from build123d import *

# Parameters (mm, degrees)
SKETCH2_W                     = 342.9
SKETCH2_H                     = 431.8
BASE_DEPTH                    = 25.4
CUT_EXTRUDE3_REACH            = 27.4
NC_POCKET_DEPTH               = 16.51
FILLET9_R                     = 6.35
FILLET6_R                     = 6.35
CBORE_FOR_M4_SHCS1_AT_2_COUNT = 2
CBORE_FOR_M4_SHCS1_AT_2_PITCH = 192.024
CBORE_FOR_M4_SHCS1_AT_3_COUNT = 2
CBORE_FOR_M4_SHCS1_AT_3_PITCH = 313.675937134
CBORE_FOR_M4_SHCS1_AT_4_COUNT = 2
CBORE_FOR_M4_SHCS1_AT_4_PITCH = 253.241439295
CBORE_FOR_M4_SHCS1_AT_5_COUNT = 2
CBORE_FOR_M4_SHCS1_AT_5_PITCH = 135.860323862
SKETCH18_R                    = 7.1755
CUT_EXTRUDE4_DEPTH            = 1.016
F_3_8_16_TAPPED_HOLE1_D       = 7.9375
F_3_8_16_TAPPED_HOLE1_DEPTH   = 27.94
F_3_8_16_TAPPED_HOLE1_TIP     = 2.384665582
F_3_8_16_TAPPED_HOLE2_D       = 7.9375
F_3_8_16_TAPPED_HOLE2_DEPTH   = 20.32
F_3_8_16_TAPPED_HOLE2_TIP     = 2.384665582
CUT_EXTRUDE5_REACH            = 10.89
FILLET1_R                     = 6.35
FILLET2_R                     = 6.35
CHAMFER1_SIZE                 = 0.508
SKETCH21_W                    = 6.35
SKETCH21_H                    = 431.8
CUT_EXTRUDE6_DEPTH            = 6.35
SKETCH22_W                    = 6.35
SKETCH22_H                    = 431.8
CUT_EXTRUDE7_DEPTH            = 3.81
SKETCH23_W                    = 33.02
SKETCH23_H                    = 48.26
CUT_EXTRUDE8_DEPTH            = 10.16
FILLET10_R                    = 6.35


with BuildPart() as part:
    # Sketch2 → Base (new body)
    with BuildSketch(Plane(origin=(0, 0, 0), x_dir=(0, 0, -1), z_dir=(1, 0, 0))):
        with Locations((-44.038996764, -78.624919094)):
            Rectangle(SKETCH2_W, SKETCH2_H)
    extrude(amount=BASE_DEPTH)

    # Sketch3 → Cut-Extrude3 (cut, up to next)
    with BuildSketch(Plane(origin=(0, 0, 0), x_dir=(0, 0, -1), z_dir=(1, 0, 0)), mode=Mode.PRIVATE) as cut_extrude3_sk1:
        Polygon((-164.688996764, -25.919919094), (-164.688996764, -229.119919094), (51.211003236, -229.119919094), (51.211003236, -146.950919094), (25.811003236, -146.950919094), (25.811003236, -25.919919094), align=None)
    cut_extrude3_tool1 = extrude(cut_extrude3_sk1.sketch, amount=CUT_EXTRUDE3_REACH, mode=Mode.PRIVATE) & part.part
    add(cut_extrude3_tool1.solids().sort_by_distance((0, -130.615794, 63.91645))[0], mode=Mode.SUBTRACT)

    # Sketch4 → NC pocket (cut)
    with BuildSketch(Plane(origin=(0, 0, 0), x_dir=(0, 0, -1), z_dir=(1, 0, 0))):
        Polygon((19.461003236, -18.299919094), (-158.338996764, -18.299919094), (-158.338996764, -25.919919094), (-164.688996764, -25.919919094), (-164.688996764, -12.583714933), (-164.688996764, -3.059919094), (-215.488996764, -3.059919094), (-215.488996764, 25.515080906), (-164.688996764, 25.515080906), (-164.688996764, 86.475080906), (-215.488996764, 86.475080906), (-215.488996764, 90.285080906), (-215.488996764, 137.275080906), (-202.788996764, 137.275080906), (51.211003236, 137.275080906), (51.211003236, -15.124919094), (51.211003236, -53.859919094), (79.405003236, -82.053919094), (51.211003236, -110.247919094), (51.211003236, -136.155919094), (51.211003236, -146.950919094), (44.861003236, -146.950919094), (44.861003236, -139.330919094), (25.811003236, -139.330919094), (25.811003236, -25.919919094), (19.461003236, -25.919919094), align=None)
    extrude(amount=NC_POCKET_DEPTH, mode=Mode.SUBTRACT)

    # Fillet9
    fillet9_edges = [part.edges().sort_by_distance(p)[0] for p in [
        (8.255, -53.859919094, -51.211003236),
        (8.255, -110.247919094, -51.211003236),
    ]]
    fillet(fillet9_edges, radius=FILLET9_R)

    # Fillet6
    fillet6_edges = [part.edges().sort_by_distance(p)[0] for p in [
        (8.255, -82.053919094, -79.405003236),
    ]]
    fillet(fillet6_edges, radius=FILLET6_R)

    # Sketch10 → CBORE for M4 SHCS1 (revolve, cut)
    with BuildSketch(Plane(origin=(25.4, 124.575080906, 151.988996764), x_dir=(0, 0, -1), z_dir=(0, 1, 0))):
        Polygon((0, 0), (0, 8.89), (2.15, 8.89), (2.15, 4), (4, 4), (4, 1), (5, 0), align=None)
    cbore_for_m4_shcs1 = revolve(axis=Axis((31.75, 124.575080906, 151.988996764), (-1, 0, 0)), mode=Mode.SUBTRACT)

    # CBORE for M4 SHCS1 at 2: CBORE for M4 SHCS1 ×2
    with Locations(*[(0, 0, -i * CBORE_FOR_M4_SHCS1_AT_2_PITCH) for i in range(1, CBORE_FOR_M4_SHCS1_AT_2_COUNT)]):
        add(cbore_for_m4_shcs1, mode=Mode.SUBTRACT)

    # CBORE for M4 SHCS1 at 3: CBORE for M4 SHCS1 ×2
    with Locations(*[Vector(0, -0.790723708, -0.612173193) * (i * CBORE_FOR_M4_SHCS1_AT_3_PITCH) for i in range(1, CBORE_FOR_M4_SHCS1_AT_3_COUNT)]):
        add(cbore_for_m4_shcs1, mode=Mode.SUBTRACT)

    # CBORE for M4 SHCS1 at 4: CBORE for M4 SHCS1 ×2
    with Locations(*[Vector(0, -0.651947013, -0.758264526) * (i * CBORE_FOR_M4_SHCS1_AT_4_PITCH) for i in range(1, CBORE_FOR_M4_SHCS1_AT_4_COUNT)]):
        add(cbore_for_m4_shcs1, mode=Mode.SUBTRACT)

    # CBORE for M4 SHCS1 at 5: CBORE for M4 SHCS1 ×2
    with Locations(*[Vector(0, -0.934783581, -0.355217761) * (i * CBORE_FOR_M4_SHCS1_AT_5_PITCH) for i in range(1, CBORE_FOR_M4_SHCS1_AT_5_COUNT)]):
        add(cbore_for_m4_shcs1, mode=Mode.SUBTRACT)

    # Sketch18 → Cut-Extrude4 (cut)
    with BuildSketch(Plane.ZY.offset(-16.51)):
        with Locations((-40.035003236, 124.575080906)):
            Circle(SKETCH18_R)
        with Locations((151.988996764, 124.575080906)):
            Circle(SKETCH18_R)
        with Locations((103.728996764, -2.424919094)):
            Circle(SKETCH18_R)
        with Locations((-40.035003236, -40.524919094)):
            Circle(SKETCH18_R)
        with Locations((-40.035003236, -123.455919094)):
            Circle(SKETCH18_R)
    extrude(amount=-CUT_EXTRUDE4_DEPTH, mode=Mode.SUBTRACT)

    # 3/8-16 Tapped Hole1
    with Locations(Plane(origin=(12.7, -294.524919094, -70.261003236), x_dir=(0, 0, -1), z_dir=(0, -1, 0))):
        with Locations((0, 0), (-114.3, 0), (-228.6, 0)):
            Hole(F_3_8_16_TAPPED_HOLE1_D / 2, depth=F_3_8_16_TAPPED_HOLE1_DEPTH)
            with Locations((0, 0, -(F_3_8_16_TAPPED_HOLE1_DEPTH + F_3_8_16_TAPPED_HOLE1_TIP / 2))):  # 118° drill point
                Cone(0, F_3_8_16_TAPPED_HOLE1_D / 2, F_3_8_16_TAPPED_HOLE1_TIP, mode=Mode.SUBTRACT)

    # 3/8-16 Tapped Hole2
    with Locations(Plane.ZY):
        with Locations((188.501496764, -220.864919094), (188.501496764, -162.444919094), (-100.423503236, -220.864919094), (-100.423503236, -162.444919094)):
            Hole(F_3_8_16_TAPPED_HOLE2_D / 2, depth=F_3_8_16_TAPPED_HOLE2_DEPTH)
            with Locations((0, 0, -(F_3_8_16_TAPPED_HOLE2_DEPTH + F_3_8_16_TAPPED_HOLE2_TIP / 2))):  # 118° drill point
                Cone(0, F_3_8_16_TAPPED_HOLE2_D / 2, F_3_8_16_TAPPED_HOLE2_TIP, mode=Mode.SUBTRACT)

    # Sketch20 → Cut-Extrude5 (cut, up to next)
    with BuildSketch(Plane.ZY.offset(-16.51), mode=Mode.PRIVATE) as cut_extrude5_sk1:
        Polygon((-51.211003236, -53.859919094), (-25.811003236, -53.859919094), (-25.811003236, -110.247919094), (-51.211003236, -110.247919094), (-79.405003236, -82.053919094), align=None)
    cut_extrude5_tool1 = extrude(cut_extrude5_sk1.sketch, amount=-CUT_EXTRUDE5_REACH, mode=Mode.PRIVATE) & part.part
    add(cut_extrude5_tool1.solids().sort_by_distance((16.51, -82.053919, -46.398071))[0], mode=Mode.SUBTRACT)

    # Fillet1
    fillet1_edges = [part.edges().sort_by_distance(p)[0] for p in [
        (20.955, -25.919919094, 164.688996764),
        (12.7, -229.119919094, 164.688996764),
        (12.7, -229.119919094, -51.211003236),
        (20.955, -146.950919094, -51.211003236),
        (20.955, -25.919919094, -25.811003236),
    ]]
    fillet(fillet1_edges, radius=FILLET1_R)

    # Fillet2
    fillet2_edges = [part.edges().sort_by_distance(p)[0] for p in [
        (20.955, -82.053919094, -79.405003236),
        (20.955, -110.247919094, -51.211003236),
        (20.955, -53.859919094, -51.211003236),
    ]]
    fillet(fillet2_edges, radius=FILLET2_R)

    # Chamfer1
    chamfer1_edges = [part.edges().sort_by_distance(p)[0] for p in [
        (12.7, -146.950919094, -25.811003236),
        (20.955, -53.859919094, -25.811003236),
        (20.955, -110.247919094, -25.811003236),
        (8.255, 86.475080906, 215.488996764),
        (8.255, 86.475080906, 164.688996764),
        (8.255, 25.515080906, 164.688996764),
        (8.255, 25.515080906, 215.488996764),
        (8.255, -3.059919094, 215.488996764),
        (8.255, -3.059919094, 164.688996764),
    ]]
    chamfer(chamfer1_edges, length=CHAMFER1_SIZE)

    # Sketch21 → Cut-Extrude6 (cut)
    with BuildSketch(Plane.ZY):
        with Locations((202.788996764, -78.624919094)):
            Rectangle(SKETCH21_W, SKETCH21_H)
        with Locations((-114.711003236, -78.624919094)):
            Rectangle(SKETCH21_W, SKETCH21_H)
    extrude(amount=-CUT_EXTRUDE6_DEPTH, mode=Mode.SUBTRACT)

    # Sketch22 → Cut-Extrude7 (cut)
    with BuildSketch(Plane(origin=(25.4, 0, 0), x_dir=(0, 0, -1), z_dir=(1, 0, 0))):
        with Locations((-205.963996764, -78.624919094)):
            Rectangle(SKETCH22_W, SKETCH22_H)
        with Locations((117.886003236, -78.624919094)):
            Rectangle(SKETCH22_W, SKETCH22_H)
    extrude(amount=-CUT_EXTRUDE7_DEPTH, mode=Mode.SUBTRACT)

    # Sketch23 → Cut-Extrude8 (cut)
    with BuildSketch(Plane.ZY):
        with Locations((-67.721003236, -159.904919094)):
            Rectangle(SKETCH23_W, SKETCH23_H)
    extrude(amount=-CUT_EXTRUDE8_DEPTH, mode=Mode.SUBTRACT)

    # Fillet10
    fillet10_edges = [part.edges().sort_by_distance(p)[0] for p in [
        (5.08, -184.034919094, -84.231003236),
        (5.08, -135.774919094, -84.231003236),
    ]]
    fillet(fillet10_edges, radius=FILLET10_R)


solid = part.part
Input: part model. Units: mm. Frame: model coordinates. A direction names the side the tool comes from. Coordinates: 2 decimals unless noted, no trailing zeros. Loops run counter-clockwise (first coordinate to the right, second up) from the corner with the lowest first, then second, coordinate; pieces in that order, holes last.
(1) Section A-A on z = 15.5. Return the cut outline in (x, y), then the cut area to 3 significant figures.
(2) Section B-B on y = -92. Return the cut outline in (x, z), then the cut area to 3 significant figures.
(3) Material intervals for probe 1 along Z at (x, y) = (22.5, -192); probe 2 along Y at (x, z) = (16, 80.5); probe 3 along Z at (x, y) = (12.7, -278.75), sorted ascending.
(4) First-contact query: pin 1 Ø10 at (y, z) = (-163, -64) entering from -X; pin 2 Ø8.5 at (y, z) = (124.58, 151.99) entering from -X; pin 3 Ø3 at (y, z) = (-70.5, -114) entering from -X. Flat tips, straight axial feed; report the tip coordinate or a pass-through.
(5) Pull-direction query (Y, two-part tool) for faces 6 (the face through (8, 42, -51.211)), 7 (the face through (18, -133, -25.811)), 8 (the face through (8, 86.475, 190)); classes: released by +Y, released by -Y, zero draft, split by the parting line, or undercut.
(6) Set-up query: faces 1 (the face through (25.4, -27.6, -24.3)), 2 (the face through (21, -53.86, -38)), 3 (the face through (8, -3.06, 190)), 4 (the face through (8, -139.331, -35)), 5 (the face through (17.526, 123, -42)). Return all of +Z, -Z, +X, -X, +Y, -Y with unobstructed straight access to the full face (end or side cutting, diameter ignored); none if empty.
Data:
1. outline: (0, -294.52) - (25.4, -294.52) - (25.4, -229.12) - (0, -229.12) - close; (0, -25.92) - (25.4, -25.92) - (25.4, 137.28) - (16.51, 137.28) - (16.51, -18.3) - (0, -18.3) - close
1. area: 3,240 mm2
2. outline: (0, -127.41) - (25.4, -127.41) - (25.4, -121.06) - (21.59, -121.06) - (21.59, -114.71) - (25.4, -114.71) - (25.4, -69.46) - (0, -69.46) - (0, -111.54) - (6.35, -111.54) - (6.35, -117.89) - (0, -117.89) - close; (0, 164.69) - (25.4, 164.69) - (25.4, 202.79) - (21.59, 202.79) - (21.59, 209.14) - (25.4, 209.14) - (25.4, 215.49) - (0, 215.49) - (0, 205.96) - (6.35, 205.96) - (6.35, 199.61) - (0, 199.61) - close
2. area: 2,630 mm2
3. probe 1: z = -127.41 to -121.06, -114.71 to -51.21, 164.69 to 202.79, 209.14 to 215.49
3. probe 2: y = -294.52 to -229.12, -25.92 to -18.3
3. probe 3: z = -127.41 to -74.23, -66.29 to 40.07, 48.01 to 154.37, 162.31 to 215.49
4. pin 1: stops at x = 10.16
4. pin 2: stops at x = 17.53
4. pin 3: stops at x = 6.35
5. face 6: zero draft
5. face 7: undercut
5. face 8: released by +Y
6. face 1: +Z, -Z, +X, +Y, -Y
6. face 2: +X, -X
6. face 3: +Z, -X
6. face 4: -X, +Y
6. face 5: -X
